Check sheet for the drawn part. Datum: minimum x, y, z corner. Units: mm. A direction names the side the tool comes from. Round coordinates to 2 decimals unless told otherwise and drop trailing zeros. Loops run counter-clockwise (first coordinate to the right, second up) from the corner with the lowest first, then second, coordinate; pieces in that order, holes last.
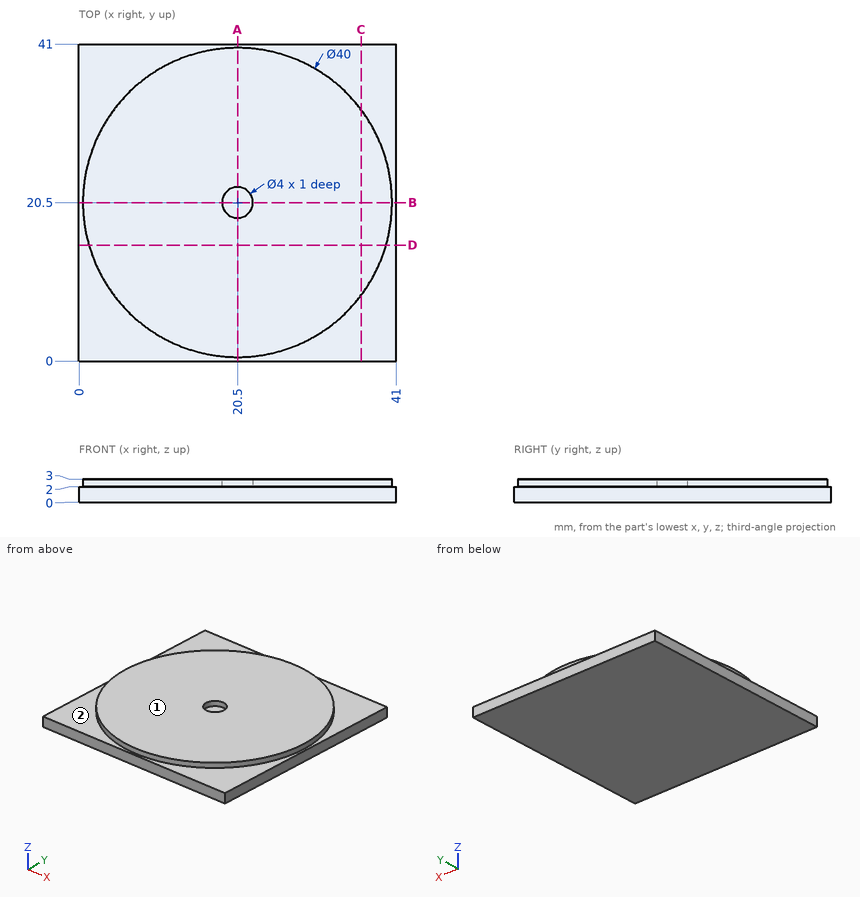
1) Sectioned sample at A-A, the plane x = 20.5. Record the cut outline in (y, z).
Report:
outline: (0, 0) - (41, 0) - (41, 2) - (40.5, 2) - (40.5, 3) - (22.5, 3) - (22.5, 2) - (18.5, 2) - (18.5, 3) - (0.5, 3) - (0.5, 2) - (0, 2) - close
2) Sectioned sample at C-C, the plane x = 36.5. Record the cut outline in (y, z), then the cut area to 3 significant figures.
Report:
outline: (0, 0) - (41, 0) - (41, 2) - (32.5, 2) - (32.5, 3) - (8.5, 3) - (8.5, 2) - (0, 2) - close
area: 106 mm2
3) Access from +Z, -Z, +X, -X, +Y, -Y to the whole of each face (thin tool, end or side, straight path). Record for the marked faces 1 and 2.
Report:
face 1: +Z, +X, -X, +Y, -Y
face 2: +Z
4) Scan lines: line 1 along Y through (x, z) = (20.5, 2.5); line 2 along Z through (x, y) = (12, 2); line 3 along X through (y, z) = (10, 2.95). Record each from-to range of solid material in increasing order.
Report:
line 1: y = 0.5 to 18.5, 22.5 to 40.5
line 2: z = 0 to 2
line 3: x = 3.48 to 37.52
5) Sectioned sample at D-D, the plane y = 15. Record the cut outline in (x, z).
Report:
outline: (0, 0) - (41, 0) - (41, 2) - (39.73, 2) - (39.73, 3) - (1.27, 3) - (1.27, 2) - (0, 2) - close
